from build123d import *

# Parameters (mm, degrees)
SKETCH1_R           = 1.27
SKETCH1_R_2         = 9.525
SKETCH1_R_3         = 3.175
BOSS_EXTRUDE1_DEPTH = 3.175
SKETCH2_W           = 76.2
SKETCH2_H           = 4.318
BOSS_EXTRUDE2_DEPTH = 54.102
BOSS_EXTRUDE3_START = 3.048
SKETCH3_W           = 76.2
SKETCH3_H           = 4.318
BOSS_EXTRUDE3_DEPTH = 3.048
SKETCH10_W          = 54.102
SKETCH10_H          = 13.716
BOSS_EXTRUDE7_DEPTH = 2.54
SKETCH5_R           = 3.429
SKETCH5_R_2         = 3.175
SKETCH5_R_3         = 1.524
SKETCH5_R_4         = 1.27
SKETCH5_R_5         = 9.779
SKETCH5_R_6         = 9.525
CUT_EXTRUDE2_DEPTH  = 76.735563806
CUT_EXTRUDE3_DEPTH  = 83.935570318
SKETCH7_R           = 12.7
CUT_EXTRUDE4_DEPTH  = 76.735563806
CUT_EXTRUDE5_DEPTH  = 99.578509321
CUT_EXTRUDE6_REACH  = 75.232
SKETCH15_R          = 2.54
CUT_EXTRUDE7_DEPTH  = 82.53914314


with BuildPart() as part:
    # Sketch1 → Boss-Extrude1 (new body)
    with BuildSketch(Plane.XY):
        Polygon((31.75, 25.4), (25.4, 25.4), (25.4, 22.86), (-25.4, 22.86), (-25.4, 25.4), (-31.75, 25.4), (-38.1, 0), (-38.1, -25.4), (38.1, -25.4), (38.1, 0), align=None)
        with Locations((-15.5448, 15.5186)):
            Circle(SKETCH1_R, mode=Mode.SUBTRACT)
        with Locations((15.4686, 15.5186)):
            Circle(SKETCH1_R, mode=Mode.SUBTRACT)
        with Locations((15.4686, -15.4678)):
            Circle(SKETCH1_R, mode=Mode.SUBTRACT)
        with Locations((-15.5448, -15.4678)):
            Circle(SKETCH1_R, mode=Mode.SUBTRACT)
        Circle(SKETCH1_R_2, mode=Mode.SUBTRACT)
        with Locations((-25.4, 0)):
            Circle(SKETCH1_R_3, mode=Mode.SUBTRACT)
        with Locations(Location((25.4, 0, 0), (0, 0, 180))):
            Circle(SKETCH1_R_3, mode=Mode.SUBTRACT)
    extrude(amount=BOSS_EXTRUDE1_DEPTH)

    # Sketch2 → Boss-Extrude2 (add)
    with BuildSketch(Plane(origin=(0, 0, 0), x_dir=(-1, 0, 0), z_dir=(0, 0, -1))):
        with Locations((0, -23.241)):
            Rectangle(SKETCH2_W, SKETCH2_H)
    extrude(amount=BOSS_EXTRUDE2_DEPTH)

    # Sketch3 → Boss-Extrude3 (add)
    with BuildSketch(Plane(origin=(0, 0, -54.102), x_dir=(-1, 0, 0), z_dir=(0, 0, -1)).offset(BOSS_EXTRUDE3_START)):
        with BuildLine():
            Line((-25.4, 6.35), (-38.1, 6.35))
            Line((-38.1, 6.35), (-38.1, -21.082))
            Line((-38.1, -21.082), (-25.4, -21.082))
            Line((-25.4, -21.082), (-25.4, -3.175))
            ThreePointArc((-25.4, -3.175), (-28.575, 0), (-25.4, 3.175))
            Line((-25.4, 3.175), (-25.4, 6.35))
        make_face()
        with BuildLine():
            Line((25.4, -3.175), (25.4, -21.082))
            Line((25.4, -21.082), (38.1, -21.082))
            Line((38.1, -21.082), (38.1, 6.35))
            Line((38.1, 6.35), (25.4, 6.35))
            Line((25.4, 6.35), (25.4, 3.175))
            ThreePointArc((25.4, 3.175), (27.64506403, 2.24506403), (28.575, 0))
            ThreePointArc((28.575, 0), (27.64506403, -2.24506403), (25.4, -3.175))
        make_face()
        with Locations((0, -23.241)):
            Rectangle(SKETCH3_W, SKETCH3_H)
    extrude(amount=-BOSS_EXTRUDE3_DEPTH)

    # Sketch10 → Boss-Extrude7 (add)
    with BuildSketch(Plane(origin=(38.1, 0, 0), x_dir=(0, 0, -1), z_dir=(1, 0, 0))):
        with Locations((27.051, -14.224)):
            Rectangle(SKETCH10_W, SKETCH10_H)
    boss_extrude7 = extrude(amount=-BOSS_EXTRUDE7_DEPTH)

    # Mirror4: Boss-Extrude7 across plane
    add(boss_extrude7.mirror(Plane(origin=(0, 0, 0), x_dir=(0, 0, 1), z_dir=(1, 0, 0))))

    # Sketch5 → Cut-Extrude2 (cut, through all)
    # profile 1 of 7: a face of its own
    with BuildSketch(Plane.XY.offset(3.175)):
        with Locations((-25.4, 0)):
            Circle(SKETCH5_R)
        with Locations((-25.4, 0)):
            Circle(SKETCH5_R_2, mode=Mode.SUBTRACT)
    # profile 2 of 7: a face of its own
    with BuildSketch(Plane.XY.offset(3.175)):
        with Locations((-15.5448, 15.5186)):
            Circle(SKETCH5_R_3)
        with Locations((-15.5448, 15.5186)):
            Circle(SKETCH5_R_4, mode=Mode.SUBTRACT)
    # profile 3 of 7: a face of its own
    with BuildSketch(Plane.XY.offset(3.175)):
        with Locations((15.4686, 15.5186)):
            Circle(SKETCH5_R_3)
        with Locations((15.4686, 15.5186)):
            Circle(SKETCH5_R_4, mode=Mode.SUBTRACT)
    # profile 4 of 7: a face of its own
    with BuildSketch(Plane.XY.offset(3.175)):
        Circle(SKETCH5_R_5)
        Circle(SKETCH5_R_6, mode=Mode.SUBTRACT)
    # profile 5 of 7: a face of its own
    with BuildSketch(Plane.XY.offset(3.175)):
        with Locations((25.4, 0)):
            Circle(SKETCH5_R)
        with Locations((25.4, 0)):
            Circle(SKETCH5_R_2, mode=Mode.SUBTRACT)
    # profile 6 of 7: a face of its own
    with BuildSketch(Plane.XY.offset(3.175)):
        with Locations((15.4686, -15.4678)):
            Circle(SKETCH5_R_3)
        with Locations((15.4686, -15.4678)):
            Circle(SKETCH5_R_4, mode=Mode.SUBTRACT)
    # profile 7 of 7: a face of its own
    with BuildSketch(Plane.XY.offset(3.175)):
        with Locations((-15.5448, -15.4678)):
            Circle(SKETCH5_R_3)
        with Locations((-15.5448, -15.4678)):
            Circle(SKETCH5_R_4, mode=Mode.SUBTRACT)
    extrude(amount=-CUT_EXTRUDE2_DEPTH, mode=Mode.SUBTRACT)

    # Sketch6 → Cut-Extrude3 (cut, through all)
    with BuildSketch(Plane(origin=(0, -21.082, 0), x_dir=(1, 0, 0), z_dir=(0, 1, 0))):
        Polygon((21.044738629, 54.102), (-21.044738629, 54.102), (0, 31.68935336), align=None)
        Polygon((-4.355261371, 27.051), (-25.4, 49.46364664), (-25.4, 4.63835336), align=None)
        Polygon((25.4, 4.63835336), (25.4, 49.46364664), (4.355261371, 27.051), align=None)
        Polygon((0, 22.41264664), (-21.044738629, 0), (21.044738629, 0), align=None)
    extrude(amount=-CUT_EXTRUDE3_DEPTH, mode=Mode.SUBTRACT)

    # Sketch7 → Cut-Extrude4 (cut, through all)
    with BuildSketch(Plane.XY.offset(3.175)):
        Circle(SKETCH7_R)
    extrude(amount=-CUT_EXTRUDE4_DEPTH, mode=Mode.SUBTRACT)

    # Sketch11 → Cut-Extrude5 (cut, through all)
    with BuildSketch(Plane(origin=(38.1, 0, 0), x_dir=(0, 0, -1), z_dir=(1, 0, 0))):
        with BuildLine():
            Line((0, -7.366), (54.102, -7.366))
            ThreePointArc((54.102, -7.366), (27.051, -17.462948896), (0, -7.366))
        make_face()
    extrude(amount=-CUT_EXTRUDE5_DEPTH, mode=Mode.SUBTRACT)

    # Sketch12 → Cut-Extrude6 (cut, up to next)
    with BuildSketch(Plane(origin=(0, 0, 0), x_dir=(-1, 0, 0), z_dir=(0, 0, -1)), mode=Mode.PRIVATE) as cut_extrude6_sk1:
        Polygon((25.4, 22.86), (16.51, 22.86), (25.4, 6.35), (38.1, 0), (31.75, 25.4), (25.4, 25.4), align=None)
    cut_extrude6_tool1 = extrude(cut_extrude6_sk1.sketch, amount=-CUT_EXTRUDE6_REACH, mode=Mode.PRIVATE) & part.part
    # Sketch12 → Cut-Extrude6 (cut, up to next)
    with BuildSketch(Plane(origin=(0, 0, 0), x_dir=(-1, 0, 0), z_dir=(0, 0, -1)), mode=Mode.PRIVATE) as cut_extrude6_sk2:
        Polygon((-25.4, 6.35), (-16.51, 22.86), (-25.4, 22.86), (-25.4, 25.4), (-31.75, 25.4), (-38.1, 0), align=None)
    cut_extrude6_tool2 = extrude(cut_extrude6_sk2.sketch, amount=-CUT_EXTRUDE6_REACH, mode=Mode.PRIVATE) & part.part
    add(cut_extrude6_tool1.solids().sort_by_distance((-28.333539, 14.25305, 0))[0], mode=Mode.SUBTRACT)
    add(cut_extrude6_tool2.solids().sort_by_distance((28.333539, 14.25305, 0))[0], mode=Mode.SUBTRACT)

    # Sketch15 → Cut-Extrude7 (cut, through all)
    with BuildSketch(Plane(origin=(0, -21.082, 0), x_dir=(1, 0, 0), z_dir=(0, 1, 0))):
        with Locations(Location((-30.988, 39.751, 0), (0, 0, 270))):
            Circle(SKETCH15_R)
        with Locations(Location((-30.988, 14.351, 0), (0, 0, 270))):
            Circle(SKETCH15_R)
        with Locations(Location((30.988, 14.351, 0), (0, 0, 90))):
            Circle(SKETCH15_R)
        with Locations(Location((30.988, 39.751, 0), (0, 0, 90))):
            Circle(SKETCH15_R)
    extrude(amount=-CUT_EXTRUDE7_DEPTH, mode=Mode.SUBTRACT)


solid = part.part
Geometry: final body of the model. Coordinates: model frame, mm. A direction names the side the tool comes from. Round coordinates to 2 decimals unless told otherwise and drop trailing zeros. Order: outer loops, then holes, each group sorted by start corner. A loop starts at its lowest first (then second) coordinate and runs counter-clockwise, first axis right, second up. Notation, with made-up numbers: (-30, 11.5) -> (16, 11.5) arc R13 cw to (16, 25.5) -> close; hole circle Ø5 at (-22.5, -36.75). An arc over 180 degrees is marked (long way). Put each result on its own line as item: value. Start each with the question number.
Q1. Section B-B on y = 8.5. Return the cut outline in (x, z) (3 decimals), and give its area (3 significant figures).
Q2. Pull-direction query (Z, two-part tool) for faces 4 (the flat face through (9, -23, -57.15)), 5 (the flat face through (-20.893, 14.721, 1.565)), 6 (the flat face through (14.73, -23.21, -16)); classes: +Z half, -Z half, draft (parallel to the pull), parting line (faces both ways), or undercut.
Q3. Reachability of faces 1 (the flat face through (25.4, 5, -56)), 2 (the flat face through (25.4, -23, -27)), 3 (the flat face through (-32, -7, -54.102)) from +Z, -Z, +X, -X, +Y, -Y: full face, straight path, thin tool, end or side. Return the list, or none.
Q4. Section A-A on z = -46.5. Return the cut outline in (x, y).
Q5. First-contact query: pin 1 (6 mm diameter, centred on x = -4.5, y = 9, fed in from -Z); pin 2 (3.5 mm diameter, centred on x = -29, z = -56.5, fed in from +Y). Flat tips, straight axial feed; report the tip coordinate or a pass-through.
Q6. Line query: probe 1 along X at (y, z) = (-8, -54); probe 2 along Z at (x, y) = (-20, -4.5) (3 decimals); probe 3 along Y at (x, z) = (3, -34). Output: solid intervals per line, ascending.
Q7. Section D-D on x = -24. Return the cut outline in (y, z) (3 decimals), and give its area (3 significant figures).
Q8. Section C-C on y = -11.5. Return the cut outline in (x, z) (3 decimals), and give its area (3 significant figures).
Ans:
1. outline: (-24.242, 0) -> (-9.436, 0) -> (-9.436, 3.175) -> (-24.242, 3.175) -> close; (9.436, 0) -> (24.242, 0) -> (24.242, 3.175) -> (9.436, 3.175) -> close
1. area: 94.0 mm2
2. face 4: -Z half
2. face 5: draft
2. face 6: undercut
3. face 1: -Z, +Y
3. face 2: +Y, -Y
3. face 3: +Y
4. outline: (-38.1, -25.4) -> (-25.4, -25.4) -> (-25.4, -21.08) -> (-35.56, -21.08) -> (-35.56, -12.59) -> (-38.1, -12.59) -> close; (-22.62, -25.4) -> (-13.91, -25.4) -> (-13.91, -21.08) -> (-22.62, -21.08) -> close; (13.91, -25.4) -> (22.62, -25.4) -> (22.62, -21.08) -> (13.91, -21.08) -> close; (25.4, -25.4) -> (38.1, -25.4) -> (38.1, -12.59) -> (35.56, -12.59) -> (35.56, -21.08) -> (25.4, -21.08) -> close
5. pin 1: stops at z = 0
5. pin 2: stops at y = 6.35
6. probe 1: x = -38.1 to -35.56, 35.56 to 38.1
6. probe 2: z = 0 to 3.175
6. probe 3: y = -25.4 to -21.08
7. outline: (-25.4, -57.15) -> (-21.082, -57.15) -> (-21.082, -47.973) -> (-25.4, -47.973) -> close; (-25.4, -6.129) -> (-21.082, -6.129) -> (-21.082, 0) -> (-3.13, 0) -> (-3.13, 3.175) -> (-25.4, 3.175) -> close; (3.13, 0) -> (8.95, 0) -> (8.95, 3.175) -> (3.13, 3.175) -> close
7. area: 155 mm2
8. outline: (-38.1, -57.15) -> (-25.4, -57.15) -> (-25.4, -54.102) -> (-35.56, -54.102) -> (-35.56, -48.424) -> (-38.1, -48.424) -> close; (-38.1, -5.678) -> (-35.56, -5.678) -> (-35.56, 0) -> (-5.389, 0) -> (-5.389, 3.175) -> (-38.1, 3.175) -> close; (5.389, 0) -> (35.56, 0) -> (35.56, -5.678) -> (38.1, -5.678) -> (38.1, 3.175) -> (5.389, 3.175) -> close; (25.4, -57.15) -> (38.1, -57.15) -> (38.1, -48.424) -> (35.56, -48.424) -> (35.56, -54.102) -> (25.4, -54.102) -> close
8. area: 343 mm2
